Geometry: see drawing. Coordinates: mm, zero at the bounding-box minimum. Round coordinates to 2 decimals unless told otherwise and drop trailing zeros. Loops run counter-clockwise (first coordinate to the right, second up) from the corner with the lowest first, then second, coordinate; pieces in that order, holes last. Notation, with made-up numbers: M 32,-28 L 68,-28 A16 cw 68,-14 Z; hole C -33,-22 d8. An arc over 180 degrees is marked long. Answer as a JSON object with one key per item and string values.
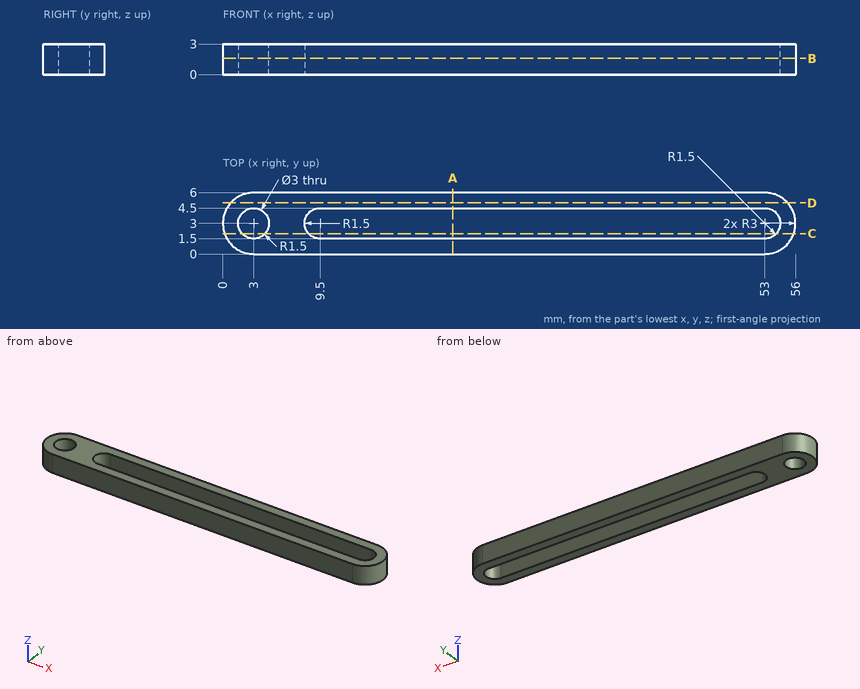
1) Pin query (flat end, axial travel): P1, Ø3.5, axis at x = 3, y = 3, coming from the +Z side; P2, Ø1.5, axis at x = 37, y = 3, coming from the +Z side. Return the tip coordinate at first contact, or that it passes through.
Results:
{"P1": "z = 3", "P2": "through"}
2) Section query B-B (z = 1.6). Return the cut outline in (x, y), and give its area (3 significant figures).
Results:
{"outline": "M 3,0 L 53,0 A3 ccw 53,6 L 3,6 A3 ccw Z; hole C 3,3 d3; hole M 9.5,1.5 L 53,1.5 A1.5 ccw 54.5,3 A1.5 ccw 53,4.5 L 9.5,4.5 A1.5 ccw Z", "area": "184 mm2"}
3) Section query D-D (y = 5). Return the cut outline in (x, z).
Results:
{"outline": "M 0.76,0 L 55.24,0 L 55.24,3 L 0.76,3 Z"}
4) Section query A-A (x = 22.5). Return the cut outline in (y, z).
Results:
{"outline": "M 0,0 L 1.5,0 L 1.5,3 L 0,3 Z; M 4.5,0 L 6,0 L 6,3 L 4.5,3 Z"}
5) Ray query, line 1 (Y direction, x = 3, z = 0.7); line 2 (X direction, y = 3.25, z = 1.1); line 3 (X direction, y = 3.5, z = 1.4). Return the intervals inside material, ascending.
Results:
{"line 1": "0 to 1.5, 4.5 to 6", "line 2": "0.01 to 1.52, 4.48 to 8.02, 54.48 to 55.99", "line 3": "0.04 to 1.59, 4.41 to 8.09, 54.41 to 55.96"}
6) Section query C-C (y = 2). Return the cut outline in (x, z), and give its area (3 significant figures).
Results:
{"outline": "M 0.17,0 L 1.88,0 L 1.88,3 L 0.17,3 Z; M 4.12,0 L 8.38,0 L 8.38,3 L 4.12,3 Z; M 54.12,0 L 55.83,0 L 55.83,3 L 54.12,3 Z", "area": "23.1 mm2"}
